from build123d import *

# Parameters (mm, degrees)
SKETCH_1_R      = 18.5
SKETCH_1_R_2    = 6.2
SKETCH_1_R_3    = 1.6
EXTRUDE_1_DEPTH = 2
CHAMFER_1_SIZE  = 0.2


with BuildPart() as part:
    # 草图1 → 凸台-拉伸1 (new body)
    with BuildSketch(Plane.XY):
        with Locations((0, -7)):
            Circle(SKETCH_1_R)
        Circle(SKETCH_1_R_2, mode=Mode.SUBTRACT)
        with Locations((15.5, -7)):
            Circle(SKETCH_1_R_3, mode=Mode.SUBTRACT)
        with Locations((7.75, -20.423393759)):
            Circle(SKETCH_1_R_3, mode=Mode.SUBTRACT)
        with Locations((-7.75, -20.423393759)):
            Circle(SKETCH_1_R_3, mode=Mode.SUBTRACT)
        with Locations((-15.5, -7)):
            Circle(SKETCH_1_R_3, mode=Mode.SUBTRACT)
        with Locations((-7.75, 6.423393759)):
            Circle(SKETCH_1_R_3, mode=Mode.SUBTRACT)
        with Locations((7.75, 6.423393759)):
            Circle(SKETCH_1_R_3, mode=Mode.SUBTRACT)
    extrude(amount=EXTRUDE_1_DEPTH)

    # 倒角1
    chamfer_1_edges = [part.edges().sort_by_distance(p)[0] for p in [
        (-18.5, -7, 0),
        (-18.5, -7, 2),
    ]]
    chamfer(chamfer_1_edges, length=CHAMFER_1_SIZE)


solid = part.part
Here's how the part is built. I have some questions about the finished solid (model axes, mm). Give positions to 0.01 mm unless a question says otherwise; leave off trailing zeros. Loops run counter-clockwise (first coordinate to the right, second up) from the corner with the lowest first, then second, coordinate; pieces in that order, holes last. Notation, with made-up numbers: (11.5, 44.25) -> (27.5, 44.25) arc R23 cw to (27.5, 63.25) -> close; hole circle Ø3 at (33.5, -2). An arc over 180 degrees is marked (long way). Answer as a JSON object with one key per item and string values. Group by question number.
Item 1: Imagine slicing it at C-C on x = 7.75. Give the number of separate pieces and of enclosed holes in the cut face, then the cut area to 3 significant figures.
Item 2: Imagine slicing it at A-A on x = 0. Write out the boundary of the cut face in (y, z), then the cut area to 3 significant figures.
Item 3: I need wall thicknesses on L1, parallel to Y at x = 7.5, z = 1.7; L2, parallel to Y at x = 7.75, z = 1.3; L3, parallel to X at y = -20, z = 0.95. Which ranges of each line are inside material? Lowest first, please.
Item 4: Imagine slicing it at B-B on z = 0.5. Write out the boundary of the cut face in (x, y).
Item 5: Will this pin go through, and if not, where does the flat tip stop? pin 1 (1.9 mm diameter, centred on x = -7.75, y = -20.42, fed in from -Z).
Answer list:
{
 "1": {"separate pieces": "3", "enclosed holes": "0", "area": "54.3 mm2"},
 "2": {"outline": "(-25.5, 0.2) -> (-25.3, 0) -> (-6.2, 0) -> (-6.2, 2) -> (-25.3, 2) -> (-25.5, 1.8) -> close; (6.2, 0) -> (11.3, 0) -> (11.5, 0.2) -> (11.5, 1.8) -> (11.3, 2) -> (6.2, 2) -> close", "area": "49.1 mm2"},
 "3": {"L1": "y = -23.91 to -22, -18.84 to 4.84, 8 to 9.91", "L2": "y = -23.8 to -22.02, -18.82 to 4.82, 8.02 to 9.8", "L3": "x = -13.16 to -9.29, -6.21 to 6.21, 9.29 to 13.16"},
 "4": {"outline": "circle Ø37 at (0, -7); hole circle Ø3.2 at (-15.5, -7); hole circle Ø3.2 at (-7.75, -20.42); hole circle Ø3.2 at (-7.75, 6.42); hole circle Ø12.4 at (0, 0); hole circle Ø3.2 at (7.75, -20.42); hole circle Ø3.2 at (7.75, 6.42); hole circle Ø3.2 at (15.5, -7)"},
 "5": {"pin 1": "passes through"}
}
